For this review, use the dimensioned drawing (mm, ordinates from the lowest corner) and the shaded views. A direction names the side the tool comes from. Coordinates: 2 decimals unless noted, no trailing zeros. Loops run counter-clockwise (first coordinate to the right, second up) from the corner with the lowest first, then second, coordinate; pieces in that order, holes last. Notation, with made-up numbers: M 39,60 L 90,60 A20 ccw 90,65 Z; hole C 83,87.25 d7. An arc over 180 degrees is marked long. Write each question's results on one line, items separated by ' | '. Start each with the question number.
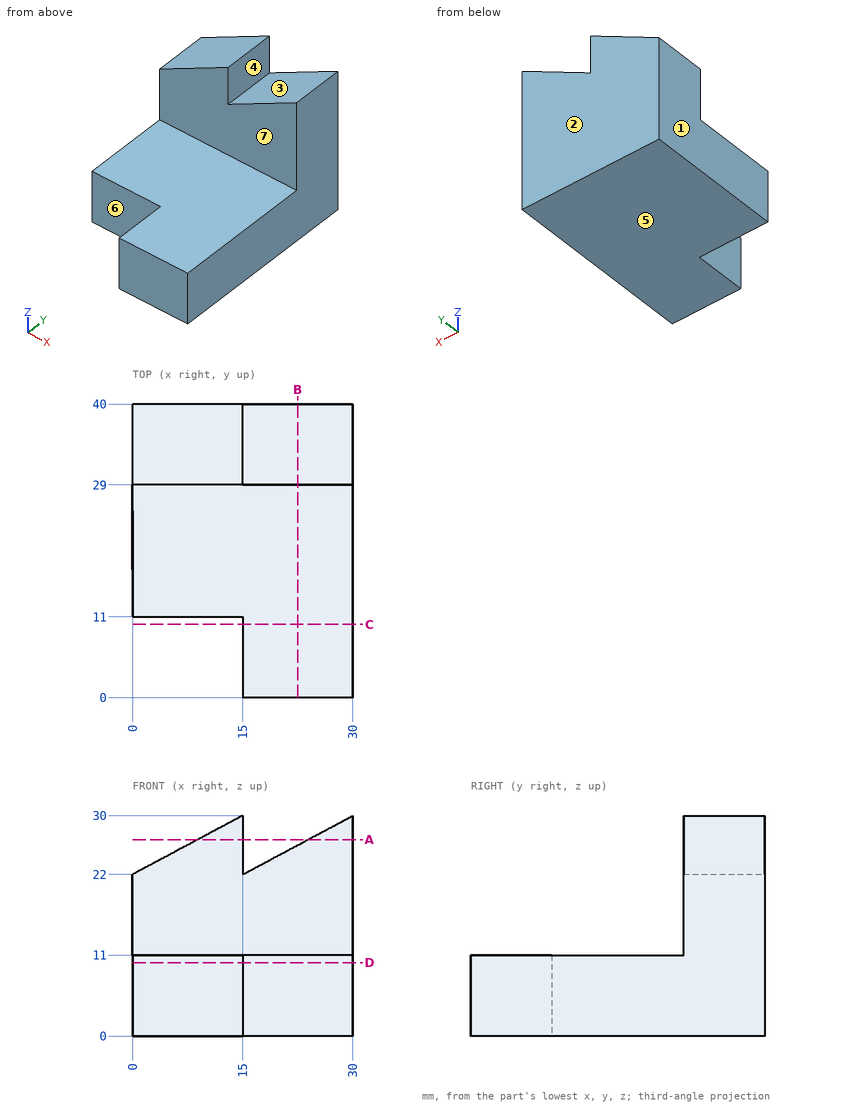
Q1. Take a section at D-D, the plane z = 10. Give the boundary of the cut face in (x, y), then the cut area to 4 significant figures.
Q2. The part is to be moulded in two halves that separate along X. For the marked faces 1, 2, 3 and 4, say which applies: pulls with the +X half, pulls with the -X half, needs draft (parallel to the pull), parting line crosses it, or undercut.
Q3. For the marked faces 5, 6 and 7, list the 3-axis set-ups (+Z, -Z, +X, -X, +Y, -Y) from which the entire face can be reached by the end or side of a thin tool; tool diameter is ignored.
Q4. Insertion check: P1, Ø12, axis at y = 3, z = 3, coming from the -X side; P2, Ø9, axis at x = 10, z = 5.5, coming from the -Y side; P3, Ø9.5, axis at x = 9, z = 19.5, coming from the -Y side. Each pin has a flat end and moves straight along its axis. Give the tip position at first contact, or say it passes through.
Q5. To check wall thickness, follow line 1 along Z through (x, y) = (19.5, 6); line 2 along Y through (x, z) = (4, 21.75); line 3 along X through (y, z) = (30, 26). State the ranges of each line that lie inside material, in increasing order.
Q6. Take a section at B-B, the plane x = 22.5. Give the boundary of the cut face in (y, z), then the cut area to 3 significant figures.
Q7. Take a section at A-A, the plane z = 26.75. Give the boundary of the cut face in (x, y).
Q8. Take a section at C-C, the plane y = 10. Give the boundary of the cut face in (x, z), then the cut area to 3 significant figures.
Results:
1) outline: M 0,11 L 15,11 L 15,0 L 30,0 L 30,40 L 0,40 Z | area: 1,035 mm^2
2) face 1: pulls with the -X half | face 2: needs draft | face 3: undercut | face 4: undercut
3) face 5: -Z, +X, -X, +Y, -Y | face 6: +Z, -Z, -X, -Y | face 7: +Z, +X, -X, -Y
4) P1: x = 15 | P2: y = 11 | P3: y = 29
5) line 1: 0 to 11 | line 2: 29 to 40 | line 3: 7.5 to 15, 22.5 to 30
6) outline: M 0,0 L 40,0 L 40,26 L 29,26 L 29,11 L 0,11 Z | area: 605 mm^2
7) outline: M 8.91,29 L 15,29 L 15,40 L 8.91,40 Z; M 23.91,29 L 30,29 L 30,40 L 23.91,40 Z
8) outline: M 15,0 L 30,0 L 30,11 L 15,11 Z | area: 165 mm^2
